Verification items for this drawing (mm, ordinates from the low corner). A direction names the side the tool comes from. Round coordinates to 2 decimals unless told otherwise and drop trailing zeros. Loops run counter-clockwise (first coordinate to the right, second up) from the corner with the lowest first, then second, coordinate; pieces in that order, holes last. Notation, with made-up numbers: (54.25, -31.5) -> (66.25, -31.5) arc R30 cw to (66.25, -6.5) -> close; hole circle Ø4 at (-22, 8). An arc over 180 degrees is marked (long way). One line per item, written item: value. Start each with the question number.
1. Material ranges on L1, parallel to X at y = 19.05, z = 18; L2, parallel to Y at x = 133, z = 29; L3, parallel to Y at x = 19, z = 10.5, recorded low to high.
2. Cross-section at C-C on x = 133.35. Record the cut outline in (y, z) (3 decimals), then the cut area to 3 significant figures.
3. Cross-section at B-B on y = 43. Record the cut outline in (x, z), then the cut area to 3 significant figures.
4. Release check for a two-part mould opening along Z. For the marked faces 1, 2 and 3 record: +Z half, -Z half, draft (parallel to the pull), parting line (faces both ways), or undercut.
5. Set-up check for the marked faces 4, 5 and 6: record each of +Z, -Z, +X, -X, +Y, -Y from which the full face is reachable in a straight line by a thin tool's end or side.
6. Go/stop test with flat-tipped pins: pin 1 (8 mm diameter, centred on x = 113.5, y = 49, fed in from -Z); pin 2 (1.5 mm diameter, centred on x = 111.5, y = 78, fed in from -Z). Record where each tip stops, or that it passes through.
7. Cross-section at D-D on y = 19.05. Record the cut outline in (x, z), then the cut area to 3 significant figures.
8. Cross-section at A-A on z = 42. Record the cut outline in (x, y) (3 decimals).
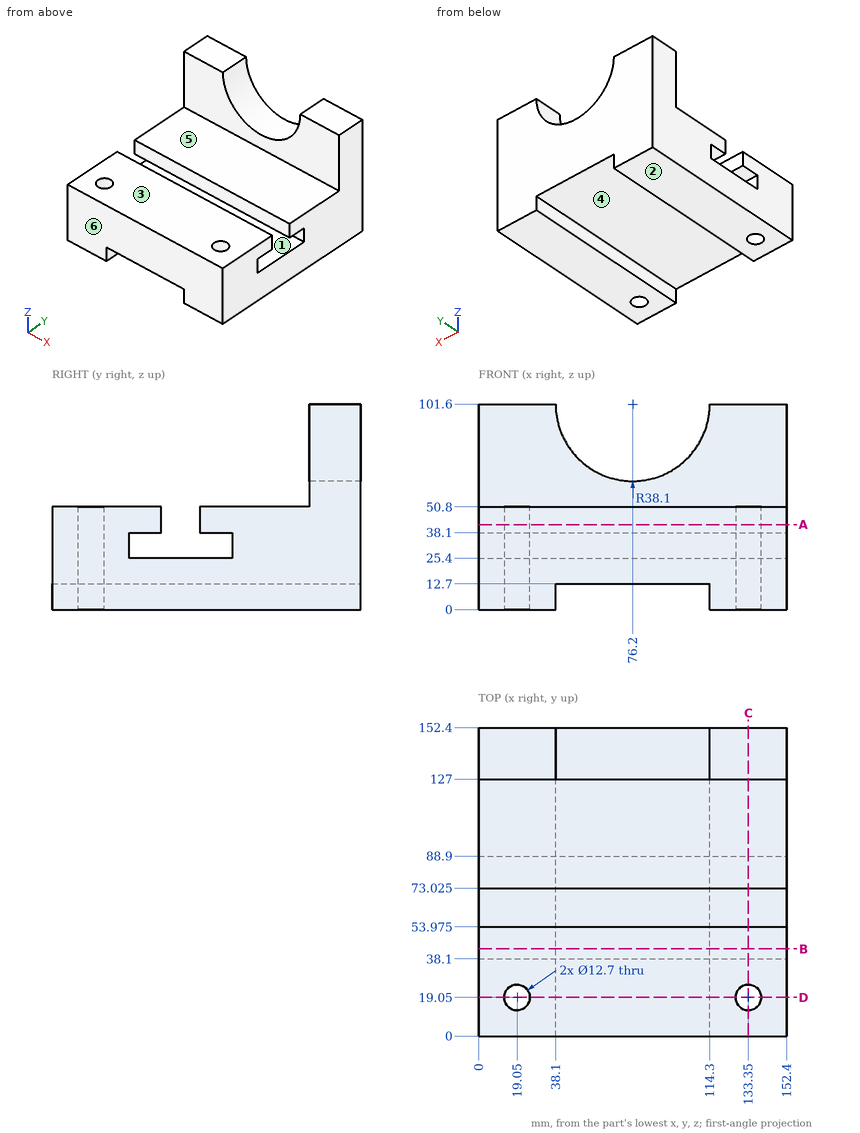
Taken from the geometry:
1. L1: x = 0 to 12.7, 25.4 to 127, 139.7 to 152.4
1. L2: y = 0 to 12.71, 25.39 to 38.1, 88.9 to 152.4
1. L3: y = 0 to 12.7, 25.4 to 152.4
2. outline: (0, 0) -> (12.7, 0) -> (12.7, 50.8) -> (0, 50.8) -> close; (25.4, 0) -> (152.4, 0) -> (152.4, 101.6) -> (127, 101.6) -> (127, 50.8) -> (73.025, 50.8) -> (73.025, 38.1) -> (88.9, 38.1) -> (88.9, 25.4) -> (38.1, 25.4) -> (38.1, 38.1) -> (53.975, 38.1) -> (53.975, 50.8) -> (25.4, 50.8) -> close
2. area: 7,500 mm2
3. outline: (0, 0) -> (38.1, 0) -> (38.1, 12.7) -> (114.3, 12.7) -> (114.3, 0) -> (152.4, 0) -> (152.4, 25.4) -> (0, 25.4) -> close; (0, 38.1) -> (152.4, 38.1) -> (152.4, 50.8) -> (0, 50.8) -> close
3. area: 4,840 mm2
4. face 1: undercut
4. face 2: -Z half
4. face 3: +Z half
5. face 4: -Z, +Y, -Y
5. face 5: +Z, +X, -X, -Y
5. face 6: +Z, -Z, +X, -X, -Y
6. pin 1: stops at z = 0
6. pin 2: stops at z = 12.7
7. outline: (0, 0) -> (12.7, 0) -> (12.7, 50.8) -> (0, 50.8) -> close; (25.4, 0) -> (38.1, 0) -> (38.1, 12.7) -> (114.3, 12.7) -> (114.3, 0) -> (127, 0) -> (127, 50.8) -> (25.4, 50.8) -> close; (139.7, 0) -> (152.4, 0) -> (152.4, 50.8) -> (139.7, 50.8) -> close
7. area: 5,480 mm2
8. outline: (0, 0) -> (152.4, 0) -> (152.4, 53.975) -> (0, 53.975) -> close; (0, 73.025) -> (152.4, 73.025) -> (152.4, 152.4) -> (0, 152.4) -> close; hole circle Ø12.7 at (19.05, 19.05); hole circle Ø12.7 at (133.35, 19.05)
